```python
from build123d import *

# Parameters (mm, degrees)
F1_DEPTH = 3


with BuildPart() as f1:
    # F0 (on Top) → F1 (new body)
    with BuildSketch(Plane.XY):
        with BuildLine():
            Line((-39.892867, 0), (-57.391304, 0))
            Line((-57.391304, 0), (-57.391304, -4.045027))
            Line((-57.391304, -4.045027), (-32.494808, -8.701925))
            Line((-32.494808, -8.701925), (-30.596264, -8.701925))
            Line((-30.596264, -8.701925), (-30.596264, -11.501925))
            Line((-30.596264, -11.501925), (-57.391304, -11.501925))
            Line((-57.391304, -11.501925), (-57.391304, -14.301925))
            Line((-57.391304, -14.301925), (-30.596264, -14.301925))
            Line((-30.596264, -14.301925), (-30.596264, -17.101925))
            Line((-30.596264, -17.101925), (-57.391304, -17.101925))
            Line((-57.391304, -17.101925), (-57.391304, -19.901925))
            Line((-57.391304, -19.901925), (-31.060893, -19.901925))
            Line((-31.060893, -19.901925), (-31.060893, -22.701925))
            Line((-31.060893, -22.701925), (-56.627642, -22.701925))
            Line((-56.627642, -22.701925), (-56.627642, -25.501925))
            Line((-56.627642, -25.501925), (-31.060893, -25.501925))
            Line((-31.060893, -25.501925), (-31.060893, -28.301925))
            Line((-31.060893, -28.301925), (-56.627642, -28.301925))
            Line((-56.627642, -28.301925), (-56.627642, -31.101925))
            Line((-56.627642, -31.101925), (-31.060893, -31.101925))
            Line((-31.060893, -31.101925), (-31.060893, -33.901925))
            Line((-31.060893, -33.901925), (-56.627642, -33.901925))
            Line((-56.627642, -33.901925), (-56.627642, -36.701925))
            Line((-56.627642, -36.701925), (-31.060893, -36.701925))
            Line((-31.060893, -36.701925), (-31.060893, -39.501925))
            Line((-31.060893, -39.501925), (-56.34404, -39.501925))
            Line((-56.34404, -39.501925), (-56.34404, -42.301925))
            Line((-56.34404, -42.301925), (-31.060893, -42.301925))
            Line((-31.060893, -42.301925), (-31.060893, -45.101925))
            Line((-31.060893, -45.101925), (-56.34404, -45.101925))
            Line((-56.34404, -45.101925), (-56.34404, -46.351925))
            Line((-56.34404, -46.351925), (-56.34404, -47.601925))
            Line((-56.34404, -47.601925), (-31.060893, -47.601925))
            Line((-31.060893, -47.601925), (-31.060893, -50.401925))
            Line((-31.060893, -50.401925), (-56.34404, -50.401925))
            Line((-56.34404, -50.401925), (-56.34404, -53.201925))
            Line((-56.34404, -53.201925), (-31.060893, -53.201925))
            Line((-31.060893, -53.201925), (-31.060893, -56.001925))
            Line((-31.060893, -56.001925), (-56.627642, -56.001925))
            Line((-56.627642, -56.001925), (-56.627642, -58.801925))
            Line((-56.627642, -58.801925), (-31.060893, -58.801925))
            Line((-31.060893, -58.801925), (-31.060893, -61.601925))
            Line((-31.060893, -61.601925), (-56.627642, -61.601925))
            Line((-56.627642, -61.601925), (-56.627642, -64.401925))
            Line((-56.627642, -64.401925), (-31.060893, -64.401925))
            Line((-31.060893, -64.401925), (-31.060893, -67.201925))
            Line((-31.060893, -67.201925), (-56.627642, -67.201925))
            Line((-56.627642, -67.201925), (-56.627642, -70.001925))
            Line((-56.627642, -70.001925), (-31.060893, -70.001925))
            Line((-31.060893, -70.001925), (-31.060893, -72.801925))
            Line((-31.060893, -72.801925), (-57.391304, -72.801925))
            Line((-57.391304, -72.801925), (-57.391304, -75.601925))
            Line((-57.391304, -75.601925), (-30.596264, -75.601925))
            Line((-30.596264, -75.601925), (-30.596264, -78.401925))
            Line((-30.596264, -78.401925), (-57.391304, -78.401925))
            Line((-57.391304, -78.401925), (-57.391304, -81.201925))
            Line((-57.391304, -81.201925), (-30.596264, -81.201925))
            Line((-30.596264, -81.201925), (-30.596264, -84.001925))
            Line((-30.596264, -84.001925), (-32.494808, -84.001925))
            Line((-32.494808, -84.001925), (-57.391304, -88.658823))
            Line((-57.391304, -88.658823), (-57.391304, -92.70385))
            Line((-57.391304, -92.70385), (-39.892867, -92.70385))
            ThreePointArc((-39.892867, -92.70385), (-12.737124, -76.069348), (-1.29091, -46.351925))
            ThreePointArc((-1.29091, -46.351925), (-12.737124, -16.634502), (-39.892867, 0))
        make_face()
    extrude(amount=F1_DEPTH)


solid = f1.part
```
Can you work these out from the model? Positions are in its coordinate system, mm. A direction names the side the tool comes from. Give positions to 0.01 mm unless a question says otherwise; leave off trailing zeros. Order: outer loops, then holes, each group sorted by start corner. A loop starts at its lowest first (then second) coordinate and runs counter-clockwise, first axis right, second up. Notation, with made-up numbers: M 24.25,36.25 L 36.25,36.25 A10 cw 36.25,44.25 Z; hole C -39.5,12.5 d11. An arc over 180 degrees is marked long. Write item = value, one per line. Start each with the question number.
Q1. We'd pull the mould along Y, two halves only. Please class faces 3 (the flat face through (-57.391, -74, 1)), 4 (the flat face through (-44, -33.902, 1)), 5 (the flat face through (-49, -92.704, 1)): pulls with the +Y half, pulls with the -Y half, needs draft (parallel to the pull), parting line crosses it, or undercut.
Q2. For faces 1 (the flat face through (-30.596, -77, 1)), 2 (the flat face through (-30, -46, 0)), which set-ups out of +Z, -Z, +X, -X, +Y, -Y let a thin tool reach every point of the face, with its end or its side?
Q3. Will these pins go through, and if not, where does the flat tip stop? pin 1 Ø0.9 at (x, z) = (-31.5, 1) entering from -Y; pin 2 Ø1.5 at (x, z) = (-32, 1.5) entering from +Y; pin 3 Ø1.4 at (y, z) = (-38, 1.5) entering from -X.
Q4. Suppose I cut it at C-C (x = -15.5). Write out the boundary of the cut face in (y, z).
Q5. I need wall thicknesses on probe 1 along Y at (x, z) = (-16, 0.35); probe 2 along Y at (x, z) = (-13, 1.3); probe 3 along X at (y, z) = (-30.5, 2.4). Which ranges of each line are inside material? Lowest first, please. Write a range as [from, to].
Q6. Suppose I cut it at B-B (y = -10). Write out the boundary of the cut face in (x, z).
Q7. Suppose I cut it at A-A (x = -49). Count the separate pieces of the cut face and the enclosed holes in it, plus the area to 3 significant figures.
Check result:
q1.face_3 = needs draft
q1.face_4 = undercut
q1.face_5 = pulls with the -Y half
q2.face_1 = +Z, -Z, -X
q2.face_2 = -Z, +X, -X, +Y, -Y
q3.pin_1 = -90.19
q3.pin_2 = -2.2
q3.pin_3 = -31.06
q4.outline = M -79.12,0 L -13.58,0 L -13.58,3 L -79.12,3 Z
q5.probe_1 = [-79.62, -13.08]
q5.probe_2 = [-76.38, -16.32]
q5.probe_3 = [-56.63, -4.58]
q6.outline = M -30.6,0 L -19.43,0 L -19.43,3 L -30.6,3 Z
q7.separate_pieces = 15
q7.enclosed_holes = 0
q7.area = 142 mm2
